Could you check a few things on this drawing? It's one solid part, dimensions in mm from its lowest x, y, z. Give positions to 0.01 mm unless a question says otherwise; leave off trailing zeros. Order: outer loops, then holes, each group sorted by start corner. A loop starts at its lowest first (then second) coordinate and runs counter-clockwise, first axis right, second up. Notation, with made-up numbers: (87.25, 0.25) - (91.25, 0.25) arc R31 ccw to (91.25, 34.25) - close; hole circle Ø1 at (39.5, 60). An arc over 180 degrees is marked (long way). Put each result on its own line as item: value.
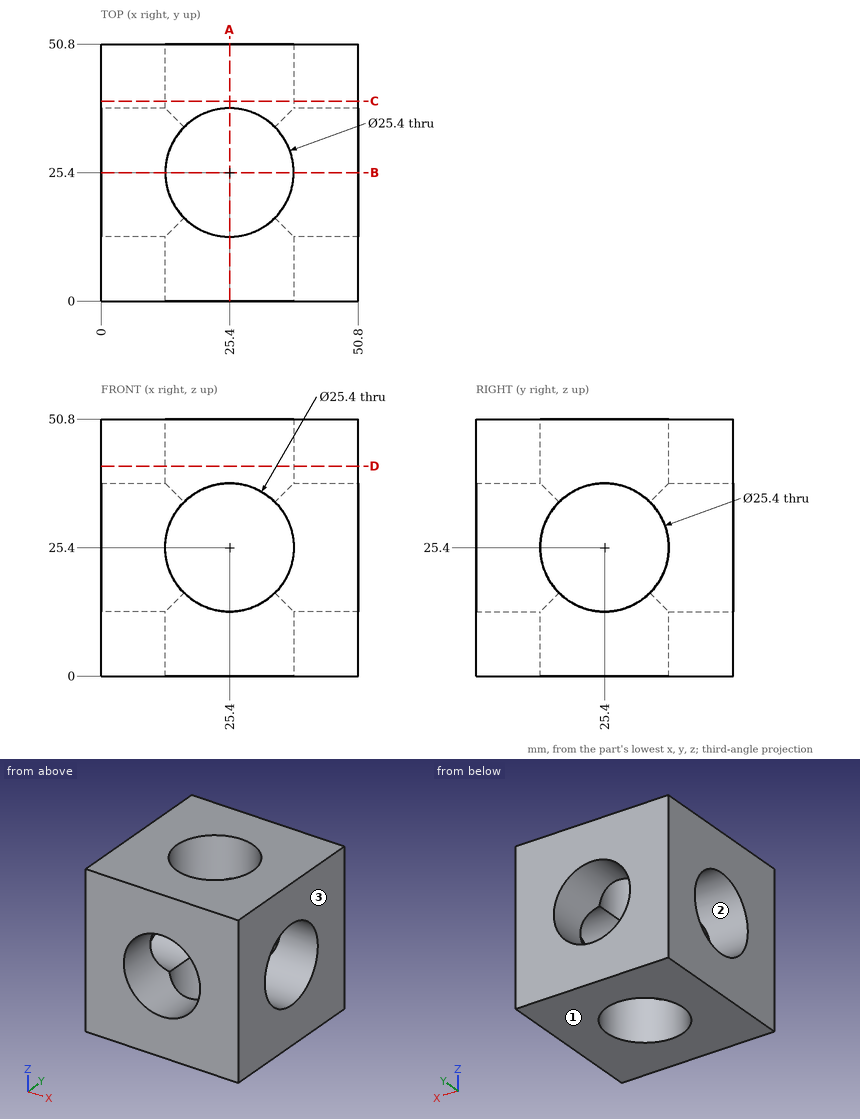
1) We'd pull the mould along Z, two halves only. Please class the marked faces 1, 2 and 3: pulls with the +Z half, pulls with the -Z half, needs draft (parallel to the pull), parting line crosses it, or undercut.
Filled in:
face 1: pulls with the -Z half
face 2: undercut
face 3: needs draft
2) Suppose I cut it at A-A, the plane x = 25.4. List the corners of the cut face in (y, z) for me, and give its area (3 significant figures).
Filled in:
outline: (0, 0) - (12.7, 0) - (12.7, 12.7) - (0, 12.7) - close; (0, 38.1) - (12.7, 38.1) - (12.7, 50.8) - (0, 50.8) - close; (38.1, 0) - (50.8, 0) - (50.8, 12.7) - (38.1, 12.7) - close; (38.1, 38.1) - (50.8, 38.1) - (50.8, 50.8) - (38.1, 50.8) - close
area: 645 mm^2
3) I'm going to push a flat-ended pin straight in: pin 1 (15 mm diameter, centred on y = 25.4, z = 25.4, fed in from +X). Where does the tip first touch, or does it pass through?
Filled in:
pin 1: passes through
4) Suppose I cut it at C-C, the plane y = 39.5. List the corners of the cut face in (x, z) for me.
Filled in:
outline: (0, 0) - (50.8, 0) - (50.8, 50.8) - (0, 50.8) - close; hole circle Ø25.4 at (25.4, 25.4)
5) If I drill on line 1 (Y direction, x = 43.5, z = 25.4); line 2 (Z direction, x = 37, y = 33), over which ranges is the centre line in solid material (lowest first)? Write a range as [from, to].
Filled in:
line 1: y = [0, 12.7], [38.1, 50.8]
line 2: z = [0, 15.23], [35.57, 50.8]
